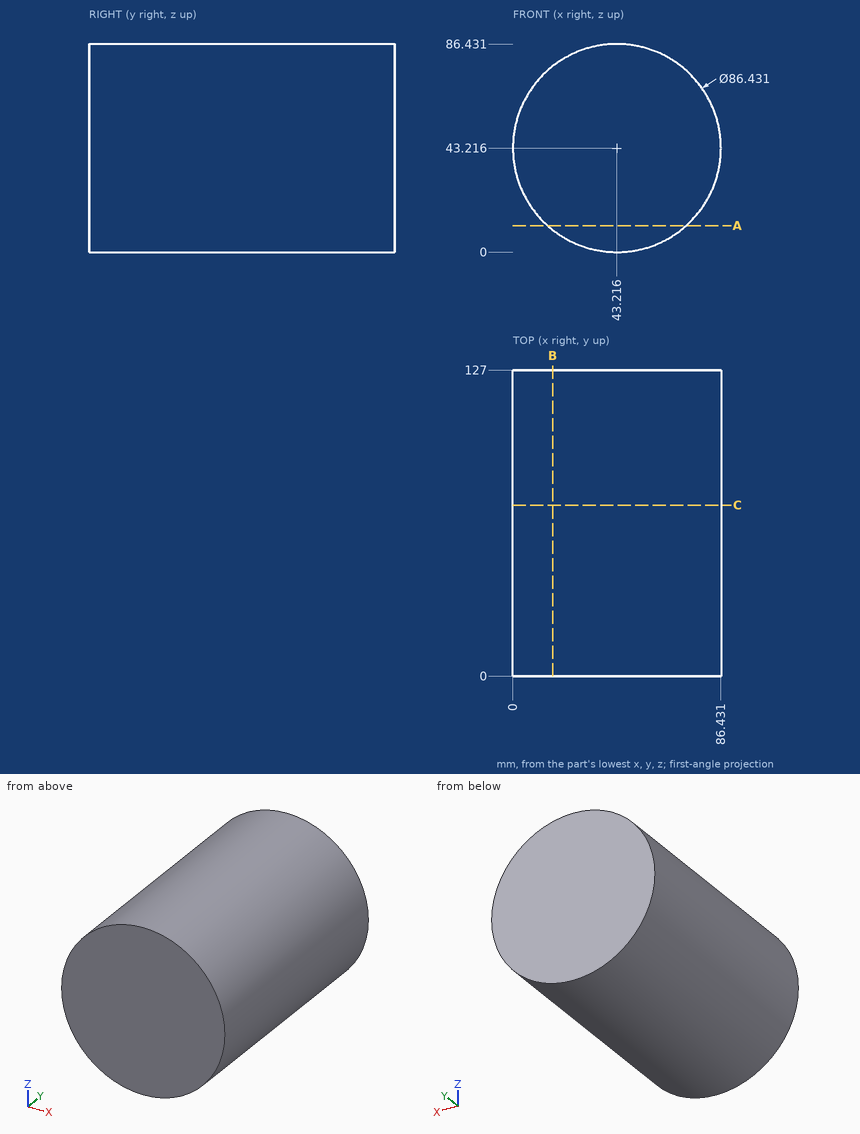
Answer from the drawing. Dimensions are ordinates in mm from the lowest x, y and z of the part. Coordinates: 2 decimals unless noted, no trailing zeros. Loops run counter-clockwise (first coordinate to the right, second up) from the corner with the lowest first, then second, coordinate; pieces in that order, holes last. Notation, with made-up numbers: (65, 84) -> (114, 84) arc R12 ccw to (114, 101) -> close; hole circle Ø3 at (79.25, -2). An arc over 180 degrees is marked (long way). Answer as CSV lines item,"result".
Q1. Each of these flat-tipped pins is pushed along its axis until it touches: pin 1 (12 mm diameter, centred on y = 51, z = 14.5, fed in from +X); pin 2 (1.5 mm diameter, centred on x = 49.5, y = 31, fed in from -Z); pin 3 (5 mm diameter, centred on y = 56, z = 70.5, fed in from +X); pin 4 (5 mm diameter, centred on x = 15, z = 77, fed in from -Y). Where does it stop, or does it pass through?
Findings:
pin 1,"stops at x = 79.98"
pin 2,"stops at z = 0.36"
pin 3,"stops at x = 78.62"
pin 4,"stops at y = 0"
Q2. The part is cut by section A-A on z = 11. Write down the section's boundary in (x, y), and give its area (3 significant figures).
Findings:
outline,"(14.41, 0) -> (72.02, 0) -> (72.02, 127) -> (14.41, 127) -> close"
area,"7,320 mm²"
Q3. The part is cut by section C-C on y = 71. Write down the section's boundary in (x, z) (1 decimal), and give its area (3 significant figures).
Findings:
outline,"circle Ø86.4 at (43.2, 43.2)"
area,"5,870 mm²"
Q4. The part is cut by section B-B on x = 16.5. Write down the section's boundary in (y, z) (1 decimal).
Findings:
outline,"(0, 9.2) -> (127, 9.2) -> (127, 77.2) -> (0, 77.2) -> close"
Q5. Find the intervals of material crossed by probe 1 along Z at (x, y) = (43.5, 55.5); probe 2 along Z at (x, y) = (34.5, 46); probe 3 along X at (y, z) = (20, 73) (1 decimal), in increasing order.
Findings:
probe 1,"z = 0 to 86.43"
probe 2,"z = 0.89 to 85.54"
probe 3,"x = 11.9 to 74.5"
